Design review of the part shown in the three views and the two pictorial views. Dimensions are in mm from the part's minimum x, y and z. A direction names the side the tool comes from. Give positions to 0.01 mm unless a question says otherwise; leave off trailing zeros. Order: outer loops, then holes, each group sorted by start corner. A loop starts at its lowest first (then second) coordinate and runs counter-clockwise, first axis right, second up.
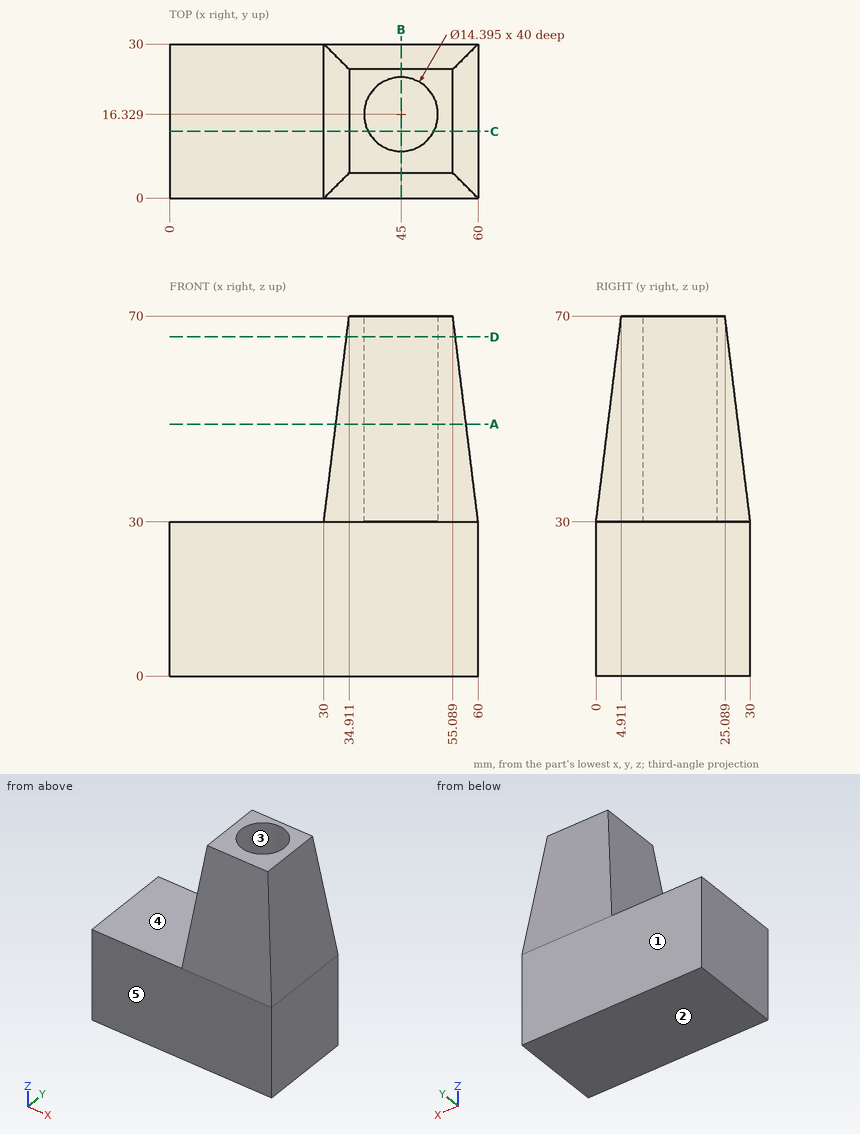
Item 1: For line 1 (Z direction, x = 18, y = 9.5); line 2 (X direction, y = 20.5, z = 30.5) (1 decimal); line 3 (Y direction, x = 45, z = 52), list the stretches that pass through material, from the lowest coordinate up.
Values found:
line 1: z = 0 to 30
line 2: x = 30.1 to 39.1, 50.9 to 59.9
line 3: y = 2.7 to 9.13, 23.53 to 27.3
Item 2: Take a section at D-D (z = 66). Give the boundary of the cut face in (x, y) (1 decimal).
Values found:
outline: (34.4, 4.4) - (55.6, 4.4) - (55.6, 25.6) - (34.4, 25.6) - close; hole circle Ø14.4 at (45, 16.3)
Item 3: Clearance check with flat-ended pins moving along their axes: pin 1 Ø8 at (x, y) = (24, 26) entering from +Z; pin 2 Ø4 at (y, z) = (25.5, 59) entering from +X (1 decimal); pin 3 Ø6 at (y, z) = (21.5, 57.5) entering from -X. State where each tip first meets the part, or that it passes through.
Values found:
pin 1: stops at z = 30
pin 2: stops at x = 56.7
pin 3: stops at x = 33.01
Item 4: Take a section at C-C (y = 13). Give the boundary of the cut face in (x, z).
Values found:
outline: (0, 0) - (60, 0) - (60, 30) - (55.09, 70) - (51.38, 70) - (51.38, 30) - (38.62, 30) - (38.62, 70) - (34.91, 70) - (30, 30) - (0, 30) - close
Item 5: Draft analysis for pull direction Y (two halves, no side actions). For the marked faces 1, 2 and 3, state which applies: released by +Y, released by -Y, zero draft, split by the parting line, or undercut.
Values found:
face 1: released by +Y
face 2: zero draft
face 3: undercut
Item 6: Take a section at B-B (x = 45). Give the boundary of the cut face in (y, z), and give its area (3 significant figures).
Values found:
outline: (0, 0) - (30, 0) - (30, 30) - (25.09, 70) - (23.53, 70) - (23.53, 30) - (9.13, 30) - (9.13, 70) - (4.91, 70) - (0, 30) - close
area: 1,330 mm2
Item 7: For the marked faces 4 and 5, list the 3-axis set-ups (+Z, -Z, +X, -X, +Y, -Y) from which the entire face can be reached by the end or side of a thin tool; tool diameter is ignored.
Values found:
face 4: +Z, -X, +Y, -Y
face 5: +Z, -Z, +X, -X, -Y
Item 8: Take a section at A-A (z = 49). Give the boundary of the cut face in (x, y) (1 decimal).
Values found:
outline: (32.3, 2.3) - (57.7, 2.3) - (57.7, 27.7) - (32.3, 27.7) - close; hole circle Ø14.4 at (45, 16.3)
